Design review of the part built by this model. Coordinates are the model's own, in mm. A direction names the side the tool comes from. Coordinates: 2 decimals unless noted, no trailing zeros. Write each loop counter-clockwise with the first axis right and the second up, starting at its lowest first coordinate (ties: lowest second). Pieces come first, ordered by that corner, then holes.
Q1. Add section D-D, the plane z = -122. Give the boundary of the cut face in (x, y) (1 decimal), plus the area to 3 significant figures.
Q2. Machinability: for faces 4 (the face through (-162, 306, -152.4)), 5 (the face through (-82.55, -9, -1)), 6 (the face through (-29, 0, -43)), 7 (the face through (-136.525, 306, 178)), which of the approach directions +Z, -Z, +X, -X, +Y, -Y give a long, thin tool a straight path to every point of the face, cutting with its end or side? Answer none if there is none.
Q3. To check wall thickness, follow probe 1 along Z at (x, y) = (0, 2.75); probe 2 along X at (y, z) = (-7, 0); probe 3 along X at (y, z) = (474, -174) (3 decimals). State the ranges of each line that lie inside material, in increasing order.
Q4. The part is to be moulded in two halves that separate along Z. For faces 1 (the face through (-140, 137, 203.2)), 2 (the face through (-58.27, -8.38, -38.67)), 3 (the face through (-136.525, -167, -178)), say which applies: +Z half, -Z half, draft (parallel to the pull), parting line (faces both ways), or undercut.
Q5. Add section A-A, the plane y = 362. Give the boundary of the cut face in (x, z) (3 decimals).
Q6. Add section B-B, the plane x = -146. Give the boundary of the cut face in (y, z).
Q7. Clearance check with flat-ended pins moving along their axes: pin 1 Ø8 at (x, z) = (59, -27) entering from +Y; pin 2 Ø19.5 at (x, y) = (32, -11.5) entering from +Z; pin 3 Ø19.5 at (y, z) = (-12, -20.5) entering from +X; pin 4 Ø12 at (x, z) = (40, -19.5) entering from -Y. State where each tip first meets the part, or that it passes through.
from build123d import *

# Parameters (mm, degrees)
BOSS_EXTRUDE2_DEPTH  = 11.1125
SKETCH1_11_W         = 50.8
SKETCH1_11_H         = 50.8
BOSS_EXTRUDE3_DEPTH  = 609.6
SKETCH1_12_W         = 50.8
SKETCH1_12_H         = 50.8
BOSS_EXTRUDE4_DEPTH  = 609.6
SKETCH1_13_W         = 50.8
SKETCH1_13_H         = 50.8
BOSS_EXTRUDE5_DEPTH  = 609.6
SKETCH1_14_W         = 50.8
SKETCH1_14_H         = 50.8
BOSS_EXTRUDE6_DEPTH  = 609.6
SKETCH4_R            = 50.8
CUT_EXTRUDE2_DEPTH   = 12.1125
SKETCH5_W            = 165.1
SKETCH5_H            = 152.4
SKETCH5_W_2          = 139.7
SKETCH5_H_2          = 127
BOSS_EXTRUDE8_DEPTH  = 17.78
SKETCH13_W           = 50.8
SKETCH13_H           = 50.8
BOSS_EXTRUDE13_DEPTH = 339.6
SKETCH15_R           = 69.931982246
SKETCH15_R_2         = 63.5
BOSS_EXTRUDE14_DEPTH = 17


with BuildPart() as part:
    # Sketch1 → Boss-Extrude2 (new body)
    with BuildSketch(Plane(origin=(0, 0, 0), x_dir=(1, 0, 0), z_dir=(0, 1, 0))):
        Polygon((-136.525, 152.4), (-187.325, 152.4), (-187.325, -203.2), (187.325, -203.2), (187.325, 203.2), (-136.525, 203.2), align=None)
    extrude(amount=BOSS_EXTRUDE2_DEPTH)

    # Sketch1<11> → Boss-Extrude3 (add)
    with BuildSketch(Plane(origin=(0, 0, 0), x_dir=(1, 0, 0), z_dir=(0, 1, 0))):
        with Locations((-161.925, 177.8)):
            Rectangle(SKETCH1_11_W, SKETCH1_11_H)
    extrude(amount=BOSS_EXTRUDE3_DEPTH)

    # Sketch1<12> → Boss-Extrude4 (add)
    with BuildSketch(Plane(origin=(0, 0, 0), x_dir=(1, 0, 0), z_dir=(0, 1, 0))):
        with Locations((-161.925, -177.8)):
            Rectangle(SKETCH1_12_W, SKETCH1_12_H)
    extrude(amount=BOSS_EXTRUDE4_DEPTH)

    # Sketch1<13> → Boss-Extrude5 (add)
    with BuildSketch(Plane(origin=(0, 0, 0), x_dir=(1, 0, 0), z_dir=(0, 1, 0))):
        with Locations((161.925, 177.8)):
            Rectangle(SKETCH1_13_W, SKETCH1_13_H)
    extrude(amount=BOSS_EXTRUDE5_DEPTH)

    # Sketch1<14> → Boss-Extrude6 (add)
    with BuildSketch(Plane(origin=(0, 0, 0), x_dir=(1, 0, 0), z_dir=(0, 1, 0))):
        with Locations((161.925, -177.8)):
            Rectangle(SKETCH1_14_W, SKETCH1_14_H)
    extrude(amount=BOSS_EXTRUDE6_DEPTH)

    # Sketch4 → Cut-Extrude2 (cut, through all)
    with BuildSketch(Plane(origin=(0, 11.1125, 0), x_dir=(1, 0, 0), z_dir=(0, 1, 0))):
        Circle(SKETCH4_R)
    extrude(amount=-CUT_EXTRUDE2_DEPTH, mode=Mode.SUBTRACT)

    # Sketch5 → Boss-Extrude8 (add)
    with BuildSketch(Plane.XZ):
        Rectangle(SKETCH5_W, SKETCH5_H)
        Rectangle(SKETCH5_W_2, SKETCH5_H_2, mode=Mode.SUBTRACT)
    extrude(amount=BOSS_EXTRUDE8_DEPTH)

    # Sketch13 → Boss-Extrude13 (add)
    with BuildSketch(Plane.XZ):
        with Locations((-161.925, 177.8)):
            Rectangle(SKETCH13_W, SKETCH13_H)
        with Locations((161.925, 177.8)):
            Rectangle(SKETCH13_W, SKETCH13_H)
        with Locations((161.925, -177.8)):
            Rectangle(SKETCH13_W, SKETCH13_H)
        with Locations((-161.925, -177.8)):
            Rectangle(SKETCH13_W, SKETCH13_H)
    extrude(amount=BOSS_EXTRUDE13_DEPTH)

    # Sketch15 → Boss-Extrude14 (add)
    with BuildSketch(Plane.XZ):
        Circle(SKETCH15_R)
        Circle(SKETCH15_R_2, mode=Mode.SUBTRACT)
    extrude(amount=BOSS_EXTRUDE14_DEPTH)


solid = part.part
Here are the results:
1. outline: (-187.3, 0) - (187.3, 0) - (187.3, 11.1) - (-187.3, 11.1) - close
1. area: 4,160 mm2
2. face 4: +X, -X, +Y
2. face 5: +Z, -Z, -X, -Y
2. face 6: -Y
2. face 7: +Z, -Z, +Y
3. probe 1: z = -203.2 to -50.8, 50.8 to 203.2
3. probe 2: x = -82.55 to -63.5, 63.5 to 82.55
3. probe 3: x = -187.325 to -136.525, 136.525 to 187.325
4. face 1: +Z half
4. face 2: undercut
4. face 3: draft
5. outline: (-187.325, -203.2) - (-136.525, -203.2) - (-136.525, -152.4) - (-187.325, -152.4) - close; (-187.325, 152.4) - (-136.525, 152.4) - (-136.525, 203.2) - (-187.325, 203.2) - close; (136.525, -203.2) - (187.325, -203.2) - (187.325, -152.4) - (136.525, -152.4) - close; (136.525, 152.4) - (187.325, 152.4) - (187.325, 203.2) - (136.525, 203.2) - close
6. outline: (-339.6, -203.2) - (609.6, -203.2) - (609.6, -152.4) - (11.11, -152.4) - (11.11, 152.4) - (609.6, 152.4) - (609.6, 203.2) - (-339.6, 203.2) - (-339.6, 152.4) - (0, 152.4) - (0, -152.4) - (-339.6, -152.4) - close
7. pin 1: stops at y = 11.11
7. pin 2: stops at z = 76.2
7. pin 3: stops at x = 82.55
7. pin 4: passes through
